The listing builds one solid part. Answer for the finished solid, in the listing's coordinates (mm). A direction names the side the tool comes from. Round coordinates to 2 decimals unless told otherwise and drop trailing zeros. Write each loop counter-clockwise with the first axis right and the second up, starting at its lowest first coordinate (ties: lowest second). Pieces come first, ordered by that corner, then holes. Notation, with made-up numbers: (1.25, 88) - (9.25, 88) arc R16 ccw to (9.25, 94) - close; hole circle Ø4 at (15, 36.25). An arc over 180 degrees is marked (long way). Answer in a Markdown table with one row per item.
from build123d import *

# Parameters (mm, degrees)
SKETCH1_W           = 215
SKETCH1_H           = 10
BOSS_EXTRUDE1_DEPTH = 5
SKETCH4_W           = 215
SKETCH4_H           = 2.5
BOSS_EXTRUDE7_DEPTH = 15
SKETCH6_W           = 215
SKETCH6_H           = 2.5
BOSS_EXTRUDE8_DEPTH = 5
SKETCH7_R           = 2.5
BOSS_EXTRUDE9_DEPTH = 10


with BuildPart() as part:
    # Sketch1 → Boss-Extrude1 (new body)
    with BuildSketch(Plane(origin=(0, 0, 0), x_dir=(1, 0, 0), z_dir=(0, 1, 0))):
        Rectangle(SKETCH1_W, SKETCH1_H)
    extrude(amount=BOSS_EXTRUDE1_DEPTH)

    # Sketch4 → Boss-Extrude7 (add)
    with BuildSketch(Plane(origin=(0, 5, 0), x_dir=(1, 0, 0), z_dir=(0, 1, 0))):
        with Locations((0, -3.75)):
            Rectangle(SKETCH4_W, SKETCH4_H)
    extrude(amount=BOSS_EXTRUDE7_DEPTH)

    # Sketch6 → Boss-Extrude8 (add)
    with BuildSketch(Plane(origin=(0, 5, 0), x_dir=(1, 0, 0), z_dir=(0, 1, 0))):
        with Locations((0, 3.75)):
            Rectangle(SKETCH6_W, SKETCH6_H)
    extrude(amount=BOSS_EXTRUDE8_DEPTH)

    # Sketch7 → Boss-Extrude9 (add)
    with BuildSketch(Plane.XY.offset(5)):
        with Locations((-97.5, 10)):
            Circle(SKETCH7_R)
        with Locations((97.5, 10)):
            Circle(SKETCH7_R)
    extrude(amount=BOSS_EXTRUDE9_DEPTH)


solid = part.part
(1) Flat-ended cylindrical pins translate along their axes: pin 1 (12 mm diameter, centred on x = 32, y = 12.5, fed in from +Z); pin 2 (3 mm diameter, centred on y = 13.5, z = 8.5, fed in from -X); pin 3 (2 mm diameter, centred on y = 10, z = 6.5, fed in from -X). Find the tip coordinate at first contact, or state that the pin passes through.
Checked values:
| item | result |
|---|---|
| pin 1 | stops at z = 5 |
| pin 2 | stops at x = -99 |
| pin 3 | stops at x = -100 |
(2) For faces 1 (the flat face through (-2, 12, 2.5)), 2 (the flat face through (97, 10, 15)), 3 (the cylindrical face through (-99, 8, 10)), determine the directions among +Z, -Z, +X, -X, +Y, -Y from which every point of the face is accessible in a straight line to the end or side of a thin tool.
Checked values:
| item | result |
|---|---|
| face 1 | +X, -X, +Y |
| face 2 | +Z, +X, -X, +Y, -Y |
| face 3 | +Z |
(3) For a pull along Z with two mould halves and no side action, classify faces 4 (the flat face through (-2, 5, 0)), 5 (the flat face through (-98, 10, 15)), 6 (the cylindrical face through (96, 8, 10)) as pulls with the +Z half, pulls with the -Z half, needs draft (parallel to the pull), parting line crosses it, or undercut.
Checked values:
| item | result |
|---|---|
| face 4 | undercut |
| face 5 | pulls with the +Z half |
| face 6 | needs draft |
(4) Section D-D (x = -97.5) is taken. Give the vertices of the cut face in (y, z).
Checked values:
| item | result |
|---|---|
| outline | (0, -5) - (10, -5) - (10, -2.5) - (5, -2.5) - (5, 2.5) - (20, 2.5) - (20, 5) - (12.5, 5) - (12.5, 15) - (7.5, 15) - (7.5, 5) - (0, 5) - close |
(5) Find the intervals of material crossed by line 1 (Z direction, x = 16, y = 6.5); line 2 (Z direction, x = 23.5, y = 10.25); line 3 (Y direction, x = 3.5, z = -2.75), in increasing order.
Checked values:
| item | result |
|---|---|
| line 1 | z = -5 to -2.5, 2.5 to 5 |
| line 2 | z = 2.5 to 5 |
| line 3 | y = 0 to 10 |
(6) Section B-B (x = 7) is taken. Give the vertices of the cut face in (y, z).
Checked values:
| item | result |
|---|---|
| outline | (0, -5) - (10, -5) - (10, -2.5) - (5, -2.5) - (5, 2.5) - (20, 2.5) - (20, 5) - (0, 5) - close |
(7) Section A-A (z = 11) is taken. Give the vertices of the cut face in (x, y), and give its area (3 significant figures).
Checked values:
| item | result |
|---|---|
| outline | circle Ø5 at (-97.5, 10); circle Ø5 at (97.5, 10) |
| area | 39.3 mm2 |
(8) Section C-C (y = 1.75) is taken. Give the vertices of the cut face in (x, z), and give its area (3 significant figures).
Checked values:
| item | result |
|---|---|
| outline | (-107.5, -5) - (107.5, -5) - (107.5, 5) - (-107.5, 5) - close |
| area | 2,150 mm2 |
